```python
from build123d import *

# Parameters (mm, degrees)
BOSS_EXTRUDE1_DEPTH = 4
SKETCH2_W           = 7
SKETCH2_H           = 5
BOSS_EXTRUDE2_DEPTH = 2
CUT_EXTRUDE1_DEPTH  = 3
BOSS_EXTRUDE3_DEPTH = 5
CUT_EXTRUDE2_DEPTH  = 15
CUT_EXTRUDE3_DEPTH  = 15


with BuildPart() as part:
    # Sketch1 → Boss-Extrude1 (new body)
    with BuildSketch(Plane.XY):
        Polygon((-3, 0.5), (-1, 2.5), (3, 2.5), (3, -2.5), (-3, -2.5), align=None)
    extrude(amount=BOSS_EXTRUDE1_DEPTH)

    # Sketch2 → Boss-Extrude2 (add)
    with BuildSketch(Plane.XZ.offset(2.5)):
        with Locations((-0.5, 2.5)):
            Rectangle(SKETCH2_W, SKETCH2_H)
    extrude(amount=-BOSS_EXTRUDE2_DEPTH)

    # Sketch3 → Cut-Extrude1 (cut)
    with BuildSketch(Plane(origin=(0, 2.5, 0), x_dir=(1, 0, 0), z_dir=(0, 1, 0))):
        Polygon((2, -4), (-3, -1.5), (-3, -4), align=None)
    extrude(amount=-CUT_EXTRUDE1_DEPTH, mode=Mode.SUBTRACT)

    # Sketch4 → Boss-Extrude3 (add)
    with BuildSketch(Plane(origin=(0, 0, 0), x_dir=(-1, 0, 0), z_dir=(0, 0, -1))):
        Polygon((-2, -0.5), (0, 1.5), (2, -0.5), (4, -0.5), (4, -2.5), (-3, -2.5), (-3, -0.5), align=None)
    extrude(amount=-BOSS_EXTRUDE3_DEPTH)

    # Sketch5 → Cut-Extrude2 (cut)
    with BuildSketch(Plane.ZY.offset(4)):
        Polygon((5, -2.5), (4, -0.5), (5, -0.5), align=None)
    extrude(amount=-CUT_EXTRUDE2_DEPTH, mode=Mode.SUBTRACT)

    # 3DSketch3 → Cut-Extrude3 (cut, along a direction that is not the sketch's normal)
    with BuildSketch(Plane(origin=(-2, -0.5, 4), x_dir=(1, 0, 0), z_dir=(0, 0.4472135954999576, 0.8944271909999162))):
        Polygon((0, 0), (2, 2.236067977), (4, 0), align=None)
    extrude(amount=CUT_EXTRUDE3_DEPTH, dir=(0, 0, 1), mode=Mode.SUBTRACT)


solid = part.part
```
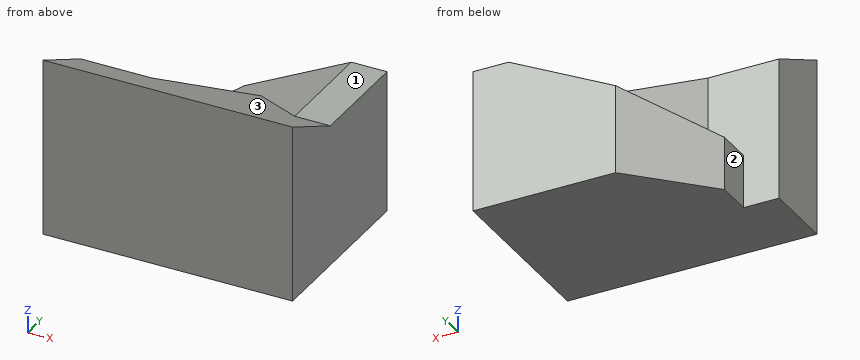
The listing builds one solid part. Answer for the finished solid, in the listing's coordinates (mm). Face numbers are marked on the shaded views. A direction names the side the tool comes from. Give positions to 0.01 mm unless a question says otherwise; leave off trailing zeros. Order: outer loops, then holes, each group sorted by start corner. A loop starts at its lowest first (then second) coordinate and runs counter-clockwise, first axis right, second up. Notation, with made-up numbers: (-24, 76) -> (25, 76) arc R30 cw to (25, 113) -> close; hole circle Ø9 at (54, 49.25). An arc over 180 degrees is marked (long way). Answer as a JSON object with one key per item and string values. Group by question number.
Item 1: Consider L1, parallel to Z at x = -2, y = 0.65; L2, parallel to Y at x = -3.5, z = 2.15; L3, parallel to X at y = 0.1, z = 1.2. Determine where each line is inside the solid, lowest interval first. Write a range as from..to.
Item 2: The part is cut by section B-B on y = 0. Write down the section's boundary in (x, z).
Item 3: The part is cut by section A-A on z = 2.85. Write down the section's boundary in (x, y).
Item 4: The part is cut by section D-D on z = 1.4. Write down the section's boundary in (x, y), and give its area (3 significant figures).
Item 5: A tool of negligible diameter and unlimited length cuts with its end or side. For the marked faces 1, 2 and 3, from which of +Z, -Z, +X, -X, +Y, -Y can it reach the whole face along a straight path? Write none if from no direction.
Item 6: The part is cut by section C-C on x = -2.5. Write down the section's boundary in (y, z), and give its area (3 significant figures).
Item 7: Flat-ended cylindrical pins translate along their axes: pin 1 (0.5 mm diameter, centred on y = 0, z = 1, fed in from -X); pin 2 (1.6 mm diameter, centred on x = -3, z = 1, fed in from +Y); pin 3 (3 mm diameter, centred on x = -3, y = 1.5, fed in from +Z). Find the tip coordinate at first contact, or state that the pin passes through.
Result set:
{
 "1": {"L1": "0..2", "L2": "-2.5..-0.5", "L3": "-3..3"},
 "2": {"outline": "(-3, 0) -> (3, 0) -> (3, 4) -> (2, 4) -> (1.5, 3.75) -> (-1.5, 3.75) -> (-1.5, 2.25) -> (-3, 1.5) -> close"},
 "3": {"outline": "(-4, -2.5) -> (3, -2.5) -> (3, 2.5) -> (-0.3, 2.5) -> (-0.3, 1.2) -> (-2, -0.5) -> (-4, -0.5) -> close"},
 "4": {"outline": "(-4, -2.5) -> (3, -2.5) -> (3, 2.5) -> (-1, 2.5) -> (-3, 0.5) -> (-3, -0.5) -> (-4, -0.5) -> close", "area": "30.0 mm²"},
 "5": {"face 1": "+Z, +X, -X, +Y", "face 2": "+Z, -Z, -X, +Y", "face 3": "+Z, -X, +Y"},
 "6": {"outline": "(-2.5, 0) -> (1, 0) -> (1, 1.75) -> (-0.5, 1.75) -> (-0.5, 4) -> (-2.5, 5) -> close", "area": "11.6 mm²"},
 "7": {"pin 1": "x = -3", "pin 2": "y = 1.3", "pin 3": "z = 2.25"}
}
